from build123d import *

# Parameters (mm, degrees)
BOSS_EXTRUDE1_DEPTH = 6
SKETCH3_W           = 30
SKETCH3_H           = 6
BOSS_EXTRUDE2_DEPTH = 6


with BuildPart() as part:
    # Sketch1 → Boss-Extrude1 (new body)
    with BuildSketch(Plane(origin=(0, 0, 0), x_dir=(1, 0, 0), z_dir=(0, 1, 0))):
        Polygon((75.5, 3), (-75.5, 3), (-69.5, -3), (69.5, -3), align=None)
    extrude(amount=BOSS_EXTRUDE1_DEPTH)

    # Sketch3 → Boss-Extrude2 (add)
    with BuildSketch(Plane.XZ):
        with Locations((50.5, -6)):
            Rectangle(SKETCH3_W, SKETCH3_H)
        with Locations((0, -6)):
            Rectangle(SKETCH3_W, SKETCH3_H)
        with Locations((-50.5, -6)):
            Rectangle(SKETCH3_W, SKETCH3_H)
    extrude(amount=-BOSS_EXTRUDE2_DEPTH)


solid = part.part
The listing builds one solid part. Answer for the finished solid, in the listing's coordinates (mm). A direction names the side the tool comes from. Give positions to 0.01 mm unless a question says otherwise; leave off trailing zeros. Write each loop counter-clockwise with the first axis right and the second up, starting at its lowest first coordinate (ties: lowest second). Pieces come first, ordered by that corner, then holes.
1) A tool of negligible diameter and unlimited length cuts with its end or side. For faces 1 (the face through (-70, 3, -3)), 2 (the face through (72.5, 3, 0)), 3 (the face through (15, 3, -6)), 4 (the face through (71, 3, -3)), from which of +Z, -Z, +X, -X, +Y, -Y can it reach the whole face along a straight path? Write none if from no direction.
2) Section C-C (x = 33) is taken. Write down the section's boundary in (y, z).
3) Given P1, Ø1.5, axis at y = 3.5, z = -6, coming from the +X side; P2, Ø4, axis at x = -28.5, z = -4.5, coming from the +Y side; P3, Ø1.8, axis at x = -70.5, y = 2.5, coming from the -Z side, each flat-ended and moving along its own axis, determine where each tip first touches the part or whether it passes through.
4) For a pull along X with two mould halves and no side action, classify faces 5 (the face through (-65.5, 3, -6)), 6 (the face through (-35.5, 3, -6)), 7 (the face through (65.5, 3, -6)), 8 (the face through (-1, 0, -2)) as pulls with the +X half, pulls with the -X half, needs draft (parallel to the pull), parting line crosses it, or undercut.
5) Find the intervals of material crossed by L1, parallel to X at y = 4.65, z = -4.5; L2, parallel to Z at x = 19, y = 0.3; L3, parallel to X at y = 0.5, z = -0.5, in increasing order.
6) Section D-D (z = 1.25) is taken. Write down the section's boundary in (x, y), and give its area (3 significant figures).
7) Section B-B (y = 3.8) is taken. Write down the section's boundary in (x, z), and give its area (3 significant figures).
8) Section A-A (z = -7.75) is taken. Write down the section's boundary in (x, y).
Response:
1. face 1: -Z, -X, +Y, -Y
1. face 2: +Z, +X, +Y, -Y
1. face 3: -Z, +Y, -Y
1. face 4: -Z, +X, +Y, -Y
2. outline: (0, -3) - (6, -3) - (6, 3) - (0, 3) - close
3. P1: stops at x = 65.5
3. P2: stops at y = 6
3. P3: stops at z = -3
4. face 5: pulls with the -X half
4. face 6: undercut
4. face 7: pulls with the +X half
4. face 8: needs draft
5. L1: x = -65.5 to -35.5, -15 to 15, 35.5 to 65.5
5. L2: z = -3 to 3
5. L3: x = -73 to 73
6. outline: (-71.25, 0) - (71.25, 0) - (71.25, 6) - (-71.25, 6) - close
6. area: 855 mm2
7. outline: (-75.5, -3) - (-65.5, -3) - (-65.5, -9) - (-35.5, -9) - (-35.5, -3) - (-15, -3) - (-15, -9) - (15, -9) - (15, -3) - (35.5, -3) - (35.5, -9) - (65.5, -9) - (65.5, -3) - (75.5, -3) - (69.5, 3) - (-69.5, 3) - close
7. area: 1,410 mm2
8. outline: (-65.5, 0) - (-35.5, 0) - (-35.5, 6) - (-65.5, 6) - close; (-15, 0) - (15, 0) - (15, 6) - (-15, 6) - close; (35.5, 0) - (65.5, 0) - (65.5, 6) - (35.5, 6) - close
